Input: dimensioned drawing with shaded views. Units: mm. Origin: part minimum x, y, z. A direction names the side the tool comes from. Round coordinates to 2 decimals unless told otherwise and drop trailing zeros. Loops run counter-clockwise (first coordinate to the right, second up) from the corner with the lowest first, then second, coordinate; pieces in that order, holes last. Notation, with made-up numbers: M 72.5,88.25 L 92.5,88.25 A17 ccw 92.5,104.25 Z; hole C 88,-39 d6. An arc over 180 degrees is marked long. Return JSON: item names as keys, results as strings.
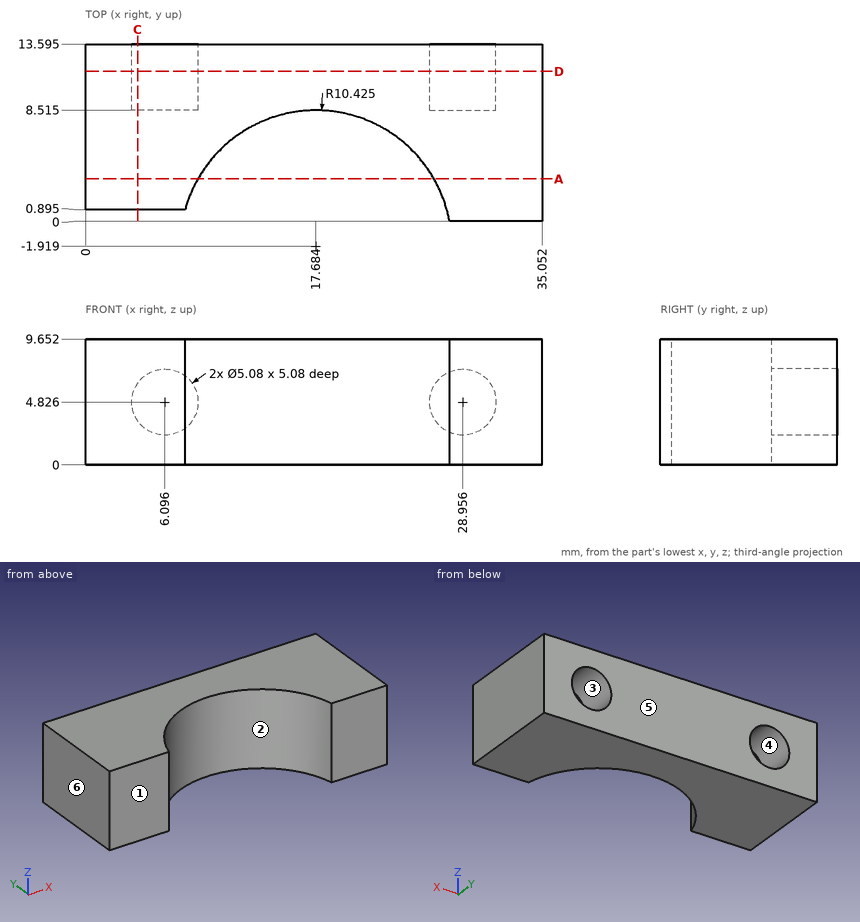
Q1. Material intervals for L1, parallel to X at y = 12.75, z = 4.25; L2, parallel to X at y = 10, z = 4.5 (1 decimal); L3, parallel to Y at x = 5.5, z = 4.5 (1 decimal), sorted ascending.
Determined:
{"L1": "x = 0 to 3.62, 8.57 to 26.48, 31.43 to 35.05", "L2": "x = 0 to 3.6, 8.6 to 26.4, 31.5 to 35.1", "L3": "y = 0.9 to 8.5"}
Q2. Section query D-D (y = 11.5). Output: boundary loops of the cut face in (x, z), plus the area to 3 significant figures.
Determined:
{"outline": "M 0,0 L 35.05,0 L 35.05,9.65 L 0,9.65 Z; hole C 6.1,4.83 d5.08; hole C 28.96,4.83 d5.08", "area": "298 mm^2"}
Q3. Pull-direction query (X, two-part tool) for the marked faces 4, 5 and 6; classes: pulls with the +X half, pulls with the -X half, needs draft (parallel to the pull), parting line crosses it, or undercut.
Determined:
{"face 4": "undercut", "face 5": "needs draft", "face 6": "pulls with the -X half"}
Q4. Pin query (flat end, axial travel): pin 1 (1.5 mm diameter, centred on x = 5, z = 4.5, fed in from +Y) (1 decimal); pin 2 (3 mm diameter, centred on y = 8.5, z = 7, fed in from -X); pin 3 (3 mm diameter, centred on x = 6.096, z = 4.826, fed in from -Y) (1 decimal). Return the tip coordinate at first contact, or that it passes through.
Determined:
{"pin 1": "stops at y = 8.5", "pin 2": "stops at x = 0", "pin 3": "stops at y = 0.9"}
Q5. Reachability of the marked faces 1, 2 and 3 from +Z, -Z, +X, -X, +Y, -Y: full face, straight path, thin tool, end or side. Return the list, or none.
Determined:
{"face 1": "+Z, -Z, -X, -Y", "face 2": "+Z, -Z, -Y", "face 3": "+Y"}
Q6. Section query C-C (x = 4). Output: boundary loops of the cut face in (y, z) (1 decimal).
Determined:
{"outline": "M 0.9,0 L 13.6,0 L 13.6,3.4 L 8.5,3.4 L 8.5,6.3 L 13.6,6.3 L 13.6,9.7 L 0.9,9.7 Z"}
Q7. Section query A-A (y = 3.25). Output: boundary loops of the cut face in (x, z).
Determined:
{"outline": "M 0,0 L 8.63,0 L 8.63,9.65 L 0,9.65 Z; M 26.74,0 L 35.05,0 L 35.05,9.65 L 26.74,9.65 Z"}
